from build123d import *

# Parameters (mm, degrees)
F0_W     = 95
F0_H     = 120
F0_W_2   = 5
F0_H_2   = 47.5
F0_W_3   = 35
F0_H_3   = 5
F1_DEPTH = 3


with BuildPart() as f1:
    # F0 (on Front) → F1 (new body)
    with BuildSketch(Plane.XZ):
        Rectangle(F0_W, F0_H)
        Polygon((37.5, -2.5), (37.5, -50), (2.5, -50), (-2.5, -50), (-37.5, -50), (-37.5, -2.5), (-37.5, 2.5), (-37.5, 50), (-2.5, 50), (2.5, 50), (37.5, 50), (37.5, 2.5), align=None, mode=Mode.SUBTRACT)
        with Locations((0, 26.25)):
            Rectangle(F0_W_2, F0_H_2)
        with Locations((0, -26.25)):
            Rectangle(F0_W_2, F0_H_2)
        with Locations((20, 0)):
            Rectangle(F0_W_3, F0_H_3)
        Rectangle(F0_W_2, F0_H_3)
        with Locations((-20, 0)):
            Rectangle(F0_W_3, F0_H_3)
    extrude(amount=F1_DEPTH)


solid = f1.part
Geometry check sheet. Reference: the model listing, model coordinates, mm. A direction names the side the tool comes from. Round coordinates to 2 decimals unless told otherwise and drop trailing zeros. Write each loop counter-clockwise with the first axis right and the second up, starting at its lowest first coordinate (ties: lowest second). Pieces come first, ordered by that corner, then holes. Notation, with made-up numbers: (48.5, 78.25) - (83.5, 78.25) arc R16 cw to (83.5, 92.25) - close; hole circle Ø1 at (44, -16.75). An arc over 180 degrees is marked (long way). One line per item, written item: value.
1. Mould release check, pull along X, two halves, no side actions. Record for faces 1 (the face through (-1, -3, 1)), 2 (the face through (-20, -1, -50)), 3 (the face through (-47.5, -1, -1)): released by +X, released by -X, zero draft, split by the parting line, or undercut.
The answers:
face 1: zero draft
face 2: undercut
face 3: released by -X
2. Depth check by flat-ended pin: pin 1 Ø10 at (x, z) = (10.5, -33) entering from +Y. Enter the tip coordinate at first touch or a pass-through.
The answers:
pin 1: passes through
3. Cross-section at B-B on x = 4.5. Record the boundary of the cut face in (y, z).
The answers:
outline: (-3, -60) - (0, -60) - (0, -50) - (-3, -50) - close; (-3, -2.5) - (0, -2.5) - (0, 2.5) - (-3, 2.5) - close; (-3, 50) - (0, 50) - (0, 60) - (-3, 60) - close
4. Set-up check for faces 4 (the face through (-1, 0, 1)), 5 (the face through (20, -1, -2.5)): record each of +Z, -Z, +X, -X, +Y, -Y from which the full face is reachable in a straight line by a thin tool's end or side.
The answers:
face 4: +Z, -Z, +X, -X, +Y
face 5: +Y, -Y
5. Scan lines: L1, parallel to X at y = -2.15, z = -21.5; L2, parallel to Z at x = -22.5, y = -2.85. Record each from-to range of solid material in increasing order.
The answers:
L1: x = -47.5 to -37.5, -2.5 to 2.5, 37.5 to 47.5
L2: z = -60 to -50, -2.5 to 2.5, 50 to 60
6. Cross-section at A-A on z = 11.5. Record the boundary of the cut face in (x, y), and give its area (3 significant figures).
The answers:
outline: (-47.5, -3) - (-37.5, -3) - (-37.5, 0) - (-47.5, 0) - close; (-2.5, -3) - (2.5, -3) - (2.5, 0) - (-2.5, 0) - close; (37.5, -3) - (47.5, -3) - (47.5, 0) - (37.5, 0) - close
area: 75.0 mm^2
7. Cross-section at C-C on y = -0.6. Record the boundary of the cut face in (x, z), and give its area (3 significant figures).
The answers:
outline: (-47.5, -60) - (47.5, -60) - (47.5, 60) - (-47.5, 60) - close; hole (-37.5, -50) - (-2.5, -50) - (-2.5, -2.5) - (-37.5, -2.5) - close; hole (-37.5, 2.5) - (-2.5, 2.5) - (-2.5, 50) - (-37.5, 50) - close; hole (2.5, -50) - (37.5, -50) - (37.5, -2.5) - (2.5, -2.5) - close; hole (2.5, 2.5) - (37.5, 2.5) - (37.5, 50) - (2.5, 50) - close
area: 4,750 mm^2
